Design review of the part built by this model. Coordinates are the model's own, in mm. Face numbers are marked on the shaded views. A direction names the side the tool comes from. Give positions to 0.01 mm unless a question says otherwise; leave off trailing zeros. Write each loop counter-clockwise with the first axis right and the second up, starting at its lowest first coordinate (ties: lowest second). Pieces come first, ordered by that corner, then holes.
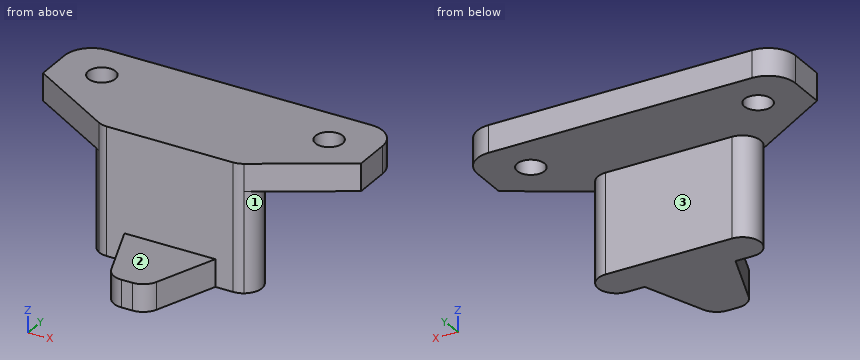
Autodesk Inventor part; units mm, degrees
ref_plane "YZ Plane" through (0, 0, 0) normal (1, 0, 0) x (0, 1, 0)
ref_plane "XZ Plane" through (0, 0, 0) normal (0, 1, 0) x (-1, 0, 0)
ref_plane "XY Plane" through (0, 0, 0) normal (0, 0, 1) x (1, 0, 0)
sketch "Sketch1" plane through (0, 0, 0) normal (0, 0, 1) x (1, 0, 0)
  line L0 (-9.4435, 4.8027) -> (25.5565, 4.8027)
  line L1 (25.5565, 4.8027) -> (25.5565, -4.1973)
  line L2 (25.5565, -4.1973) -> (-9.4435, -4.1973)
  line L3 (-9.4435, -4.1973) -> (-9.4435, 4.8027)
  line L4 (-9.4435, -4.1973) -> (-9.4435, -8.1973)
  line L5 (-9.4435, -8.1973) -> (25.5565, -8.1973)
  line L6 (25.5565, -8.1973) -> (25.5565, -4.1973)
  point P0 (0, 0)
  point P1 (-4.4435, 0.3027)
  point P2 (20.5565, 0.3027)
  dimension "d0" = 35
  dimension "d1" = 9
  dimension "d2" = 25
  dimension "d3" = 5
  dimension "d4" = 4.5
  dimension "d5" = 4
extrude "Extrusion1" add sketch "Sketch1" along normal blind 3
extrude "Extrusion2" add sketch "Sketch1" against normal blind 11 contours L2 L6 L5 L4
hole "Hole1" at (-4.4435, 0.3027, 0) at (20.5565, 0.3027, 0) direction (0, 0, 1) diameter 3 end through all
fillet "Fillet1" radius 3 2 edges at (-9.4435, 4.8027, 1.5) (25.5565, 4.8027, 1.5)
chamfer "Chamfer1" distance 6 distance2 10 1 edges at (-9.4435, -8.1973, -4) measured on face at (-9.4435, -6.8639, -2.6667)
chamfer "Chamfer2" distance 6 distance2 10 1 edges at (25.5565, -8.1973, -4) measured on face at (25.5565, -6.8639, -2.6667)
fillet "Fillet2" radius 2 4 edges at (22.2232, -4.1973, -5.5) (-6.1102, -4.1973, -5.5) (0.5565, -8.1973, -4) (15.5565, -8.1973, -4)
sketch "Sketch2" plane through (0, 0, -11) normal (0, 0, -1) x (-1, 0, 0)
  arc A0 (-15.0025, -4.1973) -> (-15.0025, -8.1973) centre (-15.0025, -6.1973) ccw
  line L0 (-15.0025, -8.1973) -> (-1.1105, -8.1973)
  arc A1 (-1.1105, -8.1973) -> (-1.1105, -4.1973) centre (-1.1105, -6.1973) ccw
  line L1 (-1.1105, -4.1973) -> (-15.0025, -4.1973)
  line L2 (-15.0025, -8.1973) -> (-1.1105, -8.1973)
  line L3 (-3.0565, -8.1973) -> (-3.0565, -16.1973)
  line L4 (-3.0565, -16.1973) -> (-13.0565, -16.1973)
  line L5 (-13.0565, -16.1973) -> (-13.0565, -8.1973)
  point P0 (0, 0)
  dimension "d25" = 8
  dimension "d26" = 10
  dimension "d27" = 13.8921
  dimension "d28" = 1.946
extrude "Extrusion3" add sketch "Sketch2" against normal blind 3 contours L0 L3 L4 L5
chamfer "Chamfer3" distance 8 distance2 3 1 edges at (3.0565, -16.1973, -9.5) measured on face at (3.0565, -13.5306, -10)
chamfer "Chamfer4" distance 8 distance2 3 1 edges at (13.0565, -16.1973, -9.5) measured on face at (13.0565, -10.8639, -10)
fillet "Fillet3" radius 2 2 edges at (10.0566, -16.1973, -9.5) (6.0564, -16.1973, -9.5)
equation "\"d1\" = 2 * d4"
equation "\"d28\" = -0.5 * d26 + 0.5 * d27"
properties part number "3DP_PLA_Y_axis_endstop_pushrod" material "ABS Plastic"
(1) Tool access review of the marked faces 1, 2 and 3: name each direction out of +Z, -Z, +X, -X, +Y, -Y from which nothing blocks a thin tool from reaching the whole face with its end or side.
Resolved:
face 1: -Z, +X
face 2: +Z, +X, -X, -Y
face 3: -Z, +X, -X, +Y
(2) Consider section D-D, the plane y = -6.25. Give the boundary of the cut face in (x, z), then the cut area to 3 significant figures.
Resolved:
outline: (-2.69, 0) - (-0.89, 0) - (-0.89, -11) - (17, -11) - (17, 0) - (18.8, 0) - (18.8, 3) - (-2.69, 3) - close
area: 261 mm2
(3) To check wall thickness, follow L1, parallel to Z at x = 10.5, y = 1; L2, parallel to X at y = -6.25, z = -6.75; L3, parallel to Y at x = 3, z = -5. State the ranges of each line that lie inside material, in increasing order.
Resolved:
L1: z = 0 to 3
L2: x = -0.89 to 17
L3: y = -8.2 to -4.2
(4) Consider section B-B, the plane x = 14. Give the boundary of the cut face in (y, z).
Resolved:
outline: (-8.2, -11) - (-4.2, -11) - (-4.2, 0) - (4.8, 0) - (4.8, 3) - (-8.2, 3) - close
(5) Consider section C-C, the plane z = 1. Give the boundary of the cut face in (x, y), then the cut area to 3 significant figures.
Resolved:
outline: (-9.44, -2.2) - (0.08, -7.91) arc R2 ccw to (1.11, -8.2) - (15, -8.2) arc R2 ccw to (16.03, -7.91) - (25.56, -2.2) - (25.56, 1.8) arc R3 ccw to (22.56, 4.8) - (-6.44, 4.8) arc R3 ccw to (-9.44, 1.8) - close; hole circle Ø3 at (-4.44, 0.3); hole circle Ø3 at (20.56, 0.3)
area: 377 mm2
(6) Clearance check with flat-ended pins moving along their axes: P1, Ø5, axis at x = -4.44, y = 0.3, coming from the +Z side; P2, Ø5.5, axis at x = 10.5, z = -3.5, coming from the +Y side; P3, Ø1, axis at x = 4.5, y = -9.5, coming from the +Z side; P4, Ø4, axis at x = 10.5, y = -1, coming from the -Z side. State where each tip first meets the part, or that it passes through.
Resolved:
P1: stops at z = 3
P2: stops at y = -4.2
P3: stops at z = -8
P4: stops at z = 0
(7) Consider section A-A, the plane y = -0.25. Give the boundary of the cut face in (x, z), then the cut area to 3 significant figures.
Resolved:
outline: (-9.44, 0) - (-5.84, 0) - (-5.84, 3) - (-9.44, 3) - close; (-3.05, 0) - (19.16, 0) - (19.16, 3) - (-3.05, 3) - close; (21.95, 0) - (25.56, 0) - (25.56, 3) - (21.95, 3) - close
area: 88.3 mm2
